Check sheet for the drawn part. Datum: minimum x, y, z corner. Units: mm. A direction names the side the tool comes from. Coordinates: 2 decimals unless noted, no trailing zeros. Order: outer loops, then holes, each group sorted by start corner. A loop starts at its lowest first (then second) coordinate and runs counter-clockwise, first axis right, second up. Notation, with made-up numbers: (-10.5, -29) -> (12.5, -29) arc R6 cw to (12.5, -18) -> close; hole circle Ø11 at (62.25, 29). An arc over 180 degrees is marked (long way). Write item = value, one per line. Start each with the question number.
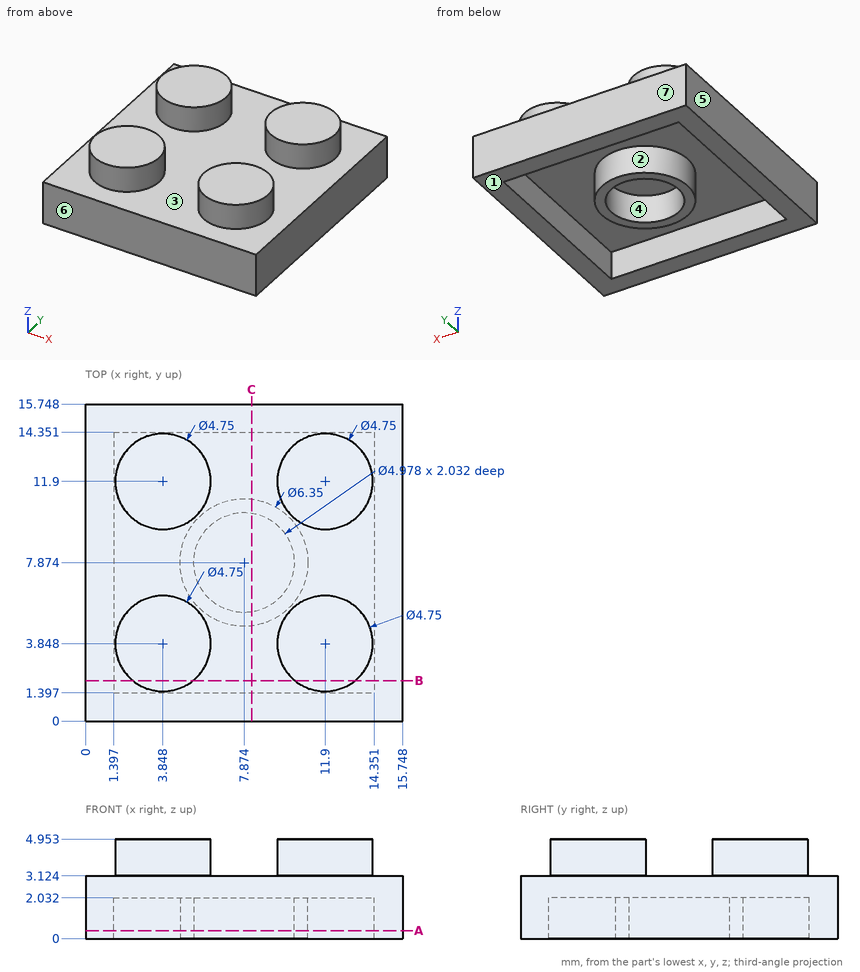
Item 1: Section check A-A (z = 0.4). State how many separate pieces and enclosed holes the cut face has.
Item 2: Gauge pin test, flat end, axial feed: P1, Ø3, axis at x = 7.874, y = 7.874, coming from the -Z side. Record the tip position at first contact, or that the pin passes through.
Item 3: Thickness scan on line 1 (X direction, y = 2.5, z = 0.55); line 2 (Y direction, x = 4, z = 4.25). Record the ranges inside material, lowest first.
Item 4: Section check B-B (y = 2). Record the boundary of the cut face in (x, z) (1 decimal).
Item 5: Section check C-C (x = 8.25). Record the boundary of the cut face in (y, z) (1 decimal).
Item 6: Tool access check on the marked faces 1, 2 and 3. Record the directions out of +Z, -Z, +X, -X, +Y, -Y that give a thin tool (end or side, any length) a straight path to the whole face; none if there is none.
Item 7: Mould release check, pull along Y, two halves, no side actions. Record for the marked faces 4, 5, 6 and 7: pulls with the +Y half, pulls with the -Y half, needs draft (parallel to the pull), parting line crosses it, or undercut.
Filled sheet:
q1.separate_pieces = 2
q1.enclosed_holes = 2
q2.P1 = 2.03
q3.line_1 = 0 to 1.4, 14.35 to 15.75
q3.line_2 = 1.48 to 6.22, 9.53 to 14.27
q4.outline = (0, 0) -> (1.4, 0) -> (1.4, 2) -> (14.4, 2) -> (14.4, 0) -> (15.7, 0) -> (15.7, 3.1) -> (13.4, 3.1) -> (13.4, 5) -> (10.4, 5) -> (10.4, 3.1) -> (5.3, 3.1) -> (5.3, 5) -> (2.4, 5) -> (2.4, 3.1) -> (0, 3.1) -> close
q5.outline = (0, 0) -> (1.4, 0) -> (1.4, 2) -> (4.7, 2) -> (4.7, 0) -> (5.4, 0) -> (5.4, 2) -> (10.3, 2) -> (10.3, 0) -> (11, 0) -> (11, 2) -> (14.4, 2) -> (14.4, 0) -> (15.7, 0) -> (15.7, 3.1) -> (0, 3.1) -> close
q6.face_1 = -Z, +X, -X, +Y, -Y
q6.face_2 = -Z
q6.face_3 = +Z
q7.face_4 = undercut
q7.face_5 = needs draft
q7.face_6 = pulls with the -Y half
q7.face_7 = pulls with the +Y half
